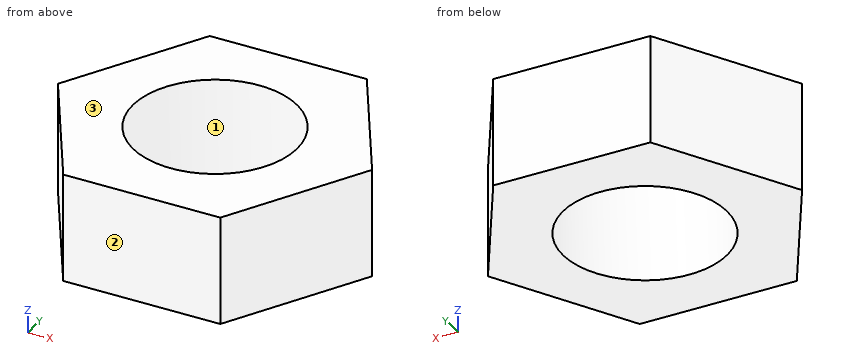
```python
from build123d import *

# Parameters (mm, degrees)
EXTRUSION1_DEPTH = 4
SKETCH2_R        = 3
THREAD1_DEPTH    = 4


with BuildPart() as part:
    # Sketch1 → Extrusion1 (new body)
    with BuildSketch(Plane.XY):
        Polygon((5.773502692, 0), (2.886751346, 5), (-2.886751346, 5), (-5.773502692, 0), (-2.886751346, -5), (2.886751346, -5), align=None)
    extrude(amount=-EXTRUSION1_DEPTH)

    # Sketch2 → Thread1 (cut)
    with BuildSketch(Plane.XY):
        Circle(SKETCH2_R)
    extrude(amount=-THREAD1_DEPTH, mode=Mode.SUBTRACT)


solid = part.part
```
Geometry check sheet. Reference: the model listing, model coordinates, mm. Face numbers are marked on the shaded views. Give positions to 0.01 mm unless a question says otherwise; leave off trailing zeros. Loops run counter-clockwise (first coordinate to the right, second up) from the corner with the lowest first, then second, coordinate; pieces in that order, holes last. Notation, with made-up numbers: M 0,-9 L 50,-9 A18 ccw 50,24 Z; hole C 12,-28 d3. An arc over 180 degrees is marked long. Write item = value, one per line.
(1) Sectioned sample at D-D, the plane x = 3.75. Record the cut outline in (y, z).
Answer below:
outline = M -3.5,-4 L 3.5,-4 L 3.5,0 L -3.5,0 Z
(2) Sectioned sample at B-B, the plane y = 1. Record the cut outline in (x, z), plus the area to 3 significant figures.
Answer below:
outline = M -5.2,-4 L -2.83,-4 L -2.83,0 L -5.2,0 Z; M 2.83,-4 L 5.2,-4 L 5.2,0 L 2.83,0 Z
area = 18.9 mm2
(3) Release check for a two-part mould opening along Y. For the marked faces 1, 2 and 3 record: released by +Y, released by -Y, zero draft, split by the parting line, or undercut.
Answer below:
face_1 = undercut
face_2 = released by -Y
face_3 = zero draft
(4) Sectioned sample at C-C, the plane z = -1. Record the cut outline in (x, y), plus the area to 3 significant figures.
Answer below:
outline = M -5.77,0 L -2.89,-5 L 2.89,-5 L 5.77,0 L 2.89,5 L -2.89,5 Z; hole C 0,0 d6
area = 58.3 mm2
(5) Material ranges on line 1 (Y direction, x = 0, z = -0.9); line 2 (X direction, y = 1.5, z = -2.85); line 3 (X direction, y = 2.25, z = -0.6), recorded low to high. Write a range as [from, to].
Answer below:
line_1 = [-5, -3], [3, 5]
line_2 = [-4.91, -2.6], [2.6, 4.91]
line_3 = [-4.47, -1.98], [1.98, 4.47]
(6) Gauge pin test, flat ends, axial feed: pin 1 Ø1.5 at (x, y) = (-1, -2.5) entering from -Z; pin 2 Ø1.5 at (y, z) = (4, -2.5) entering from +X. Record the tip position at first contact, or that the pin passes through.
Answer below:
pin_1 = -4
pin_2 = 3.9
(7) Sectioned sample at A-A, the plane x = 0. Record the cut outline in (y, z), plus the area to 3 significant figures.
Answer below:
outline = M -5,-4 L -3,-4 L -3,0 L -5,0 Z; M 3,-4 L 5,-4 L 5,0 L 3,0 Z
area = 16.0 mm2
